```python
from build123d import *

# Parameters (mm, degrees)
F0_R     = 1.5
F0_W     = 114
F0_H     = 114
F0_W_2   = 110
F0_H_2   = 110
F1_DEPTH = 2
F0_W_3   = 7
F0_H_3   = 30
F2_DEPTH = 2.5
F0_H_4   = 5
F0_W_4   = 8
F3_DEPTH = 10
F4_SIZE  = 7.99999
F5_R     = 4
F6_DEPTH = 25
F7_R     = 3
F8_R     = 5
F10_D    = 3


# Not quite as in the source:
# - a fillet or chamfer is up to 0.001 mm smaller than in the source, because OpenCascade refuses the exact size


with BuildPart() as f1:
    # F0 (on Front) → F1 (new body)
    with BuildSketch(Plane.XZ):
        with BuildLine():
            Line((-68, 17.5), (-75, 17.5))
            Line((-75, 17.5), (-75, -17.5))
            Line((-75, -17.5), (-68, -17.5))
            Line((-68, -17.5), (-68, -56.2650060048))
            ThreePointArc((-68, -56.2650060048), (-60.8578643763, -60.8578643763), (-56.2650060048, -68))
            Line((-56.2650060048, -68), (56.2650060048, -68))
            ThreePointArc((56.2650060048, -68), (60.8578643763, -60.8578643763), (68, -56.2650060048))
            Line((68, -56.2650060048), (68, -20))
            Line((68, -20), (60, -20))
            Line((60, -20), (60, -15))
            Line((60, -15), (68, -15))
            Line((68, -15), (68, 15))
            Line((68, 15), (60, 15))
            Line((60, 15), (60, 20))
            Line((60, 20), (68, 20))
            Line((68, 20), (68, 56.2650060048))
            ThreePointArc((68, 56.2650060048), (60.8578643763, 60.8578643763), (56.2650060048, 68))
            Line((56.2650060048, 68), (-56.2650060048, 68))
            ThreePointArc((-56.2650060048, 68), (-60.8578643763, 60.8578643763), (-68, 56.2650060048))
            Line((-68, 56.2650060048), (-68, 17.5))
        make_face()
        with Locations((-70, 0)):
            Circle(F0_R, mode=Mode.SUBTRACT)
        Rectangle(F0_W, F0_H, mode=Mode.SUBTRACT)
        Rectangle(F0_W, F0_H)
        Rectangle(F0_W_2, F0_H_2, mode=Mode.SUBTRACT)
    extrude(amount=F1_DEPTH)

    # F0 (on Front) → F2 (join)
    with BuildSketch(Plane.XZ):
        with BuildLine():
            Line((-68, 68), (-68, 56.2650060048))
            ThreePointArc((-68, 56.2650060048), (-60.8578643763, 60.8578643763), (-56.2650060048, 68))
            Line((-56.2650060048, 68), (-68, 68))
        make_face()
        Polygon((75, 20), (75, 75), (-75, 75), (-75, 17.5), (-68, 17.5), (-68, 56.2650060048), (-68, 68), (-56.2650060048, 68), (56.2650060048, 68), (68, 68), (68, 56.2650060048), (68, 20), align=None)
        with BuildLine():
            ThreePointArc((56.2650060048, 68), (60.8578643763, 60.8578643763), (68, 56.2650060048))
            Line((68, 56.2650060048), (68, 68))
            Line((68, 68), (56.2650060048, 68))
        make_face()
        with BuildLine():
            Line((68, -68), (68, -56.2650060048))
            ThreePointArc((68, -56.2650060048), (60.8578643763, -60.8578643763), (56.2650060048, -68))
            Line((56.2650060048, -68), (68, -68))
        make_face()
        with BuildLine():
            ThreePointArc((-56.2650060048, -68), (-60.8578643763, -60.8578643763), (-68, -56.2650060048))
            Line((-68, -56.2650060048), (-68, -68))
            Line((-68, -68), (-56.2650060048, -68))
        make_face()
        Polygon((-68, -17.5), (-75, -17.5), (-75, -75), (75, -75), (75, -20), (68, -20), (68, -56.2650060048), (68, -68), (56.2650060048, -68), (-56.2650060048, -68), (-68, -68), (-68, -56.2650060048), align=None)
        with Locations((71.5, 0)):
            Rectangle(F0_W_3, F0_H_3)
    extrude(amount=F2_DEPTH)

    # F0 (on Front) → F3 (join)
    with BuildSketch(Plane.XZ):
        with Locations((71.5, 17.5)):
            Rectangle(F0_W_3, F0_H_4)
        with Locations((64, 17.5)):
            Rectangle(F0_W_4, F0_H_4)
        with Locations((64, -17.5)):
            Rectangle(F0_W_4, F0_H_4)
        with Locations((71.5, -17.5)):
            Rectangle(F0_W_3, F0_H_4)
    extrude(amount=F3_DEPTH)

    # F4 (size 8 in the source; OpenCascade refuses exactly that, so slightly less here)
    f4_edges = [f1.edges().sort_by_distance(p)[0] for p in [
        (60, -10, 17.5),
        (60, -10, -17.5),
    ]]
    chamfer(f4_edges, length=F4_SIZE)

    # F5
    f5_edges = [f1.edges().sort_by_distance(p)[0] for p in [
        (75, -10, 17.5),
        (75, -10, -17.5),
    ]]
    fillet(f5_edges, radius=F5_R)

    # F0 (on Front) → F6 (join)
    with BuildSketch(Plane.XZ):
        Rectangle(F0_W, F0_H)
        Rectangle(F0_W_2, F0_H_2, mode=Mode.SUBTRACT)
    extrude(amount=-F6_DEPTH)

    # F7
    f7_edges = [f1.edges().sort_by_distance(p)[0] for p in [
        (-55, 11.5, 55),
        (55, 11.5, 55),
        (55, 11.5, -55),
        (-55, 11.5, -55),
    ]]
    fillet(f7_edges, radius=F7_R)

    # F8
    f8_edges = [f1.edges().sort_by_distance(p)[0] for p in [
        (57, 12.5, 57),
        (57, 12.5, -57),
        (-57, 12.5, -57),
        (-57, 12.5, 57),
        (-75, -1.25, 75),
        (-75, -1.25, -75),
        (75, -1.25, -75),
        (75, -1.25, 75),
    ]]
    fillet(f8_edges, radius=F8_R)

    # F10 (through all)
    with Locations(Plane.XY.offset(20)):
        with Locations((71, -6)):
            Hole(F10_D / 2)


solid = f1.part
```
Part model, mm, in its own coordinate system. A direction names the side the tool comes from. Coordinates: 2 decimals unless noted, no trailing zeros. Order: outer loops, then holes, each group sorted by start corner. A loop starts at its lowest first (then second) coordinate and runs counter-clockwise, first axis right, second up. Notation, with made-up numbers: (-29.5, -6.75) -> (-14.5, -6.75) arc R29 ccw to (-14.5, 23.25) -> close; hole circle Ø5 at (7, -8.5). An arc over 180 degrees is marked (long way). Put each result on its own line as item: value. Start each with the question number.
(1) Band-saw the part on A-A (x = 24). Give the cut face in (y, z).
(2) Pin check, flat tips, straight feed: pin 1 Ø2.5 at (x, y) = (71, -6.5) entering from -Z; pin 2 Ø8 at (x, y) = (25, 10) entering from +Z; pin 3 Ø6 at (x, y) = (43, 16) entering from -Z. Stop position of each tip, or through.
(3) Mould opens along X. For faces 1 (the face through (-57, 12, -1)), 2 (the face through (-55.2, 25, 25.6)), 3 (the face through (73.859, -8.797, 17.535)), 4 (the face through (60.773, -2.246, 60.943)) say: pulls with the +X half, pulls with the -X half, needs draft (parallel to the pull), parting line crosses it, or undercut.
(4) Probe line 1 along X through (y, z) = (7.5, 41.5); line 2 along Y through (x, z) = (71, 17). List the from-to ranges inside material, lowest first. Write a range as [from, to].
(5) Band-saw the part on B-B (z = -29). Give the cut face in (x, y).
(6) Which spindle directions (+Z, -Z, +X, -X, +Y, -Y) get a long thin tool onto all of the face, cutting with end or side? Do faces 5 (the face through (-60.943, -2.246, 60.773)), 6 (the face through (-56, 13, -55)), 7 (the face through (71, -2.5, 0)), 8 (the face through (-1, 11, 55)), 9 (the face through (-68, 0, 1)). Say none if no direction does.
(7) Band-saw the part on D-D (z = 59). Give the cut face in (x, y).
(8) Band-saw the part on C-C (y = 19). Give the cut face in (x, z).
Determined:
1. outline: (-2.5, -75) -> (0, -75) -> (0, -57) -> (25, -57) -> (25, -55) -> (-2, -55) -> (-2, -68) -> (-2.5, -68) -> close; (-2.5, 68) -> (-2, 68) -> (-2, 55) -> (25, 55) -> (25, 57) -> (0, 57) -> (0, 75) -> (-2.5, 75) -> close
2. pin 1: stops at z = -20
2. pin 2: stops at z = 57
2. pin 3: stops at z = -57
3. face 1: pulls with the -X half
3. face 2: needs draft
3. face 3: pulls with the +X half
3. face 4: undercut
4. line 1: x = [-57, -55], [55, 57]
4. line 2: y = [-10, -7.5], [-4.5, 0]
5. outline: (-75, -2.5) -> (-68, -2.5) -> (-68, -2) -> (-55, -2) -> (-55, 25) -> (-57, 25) -> (-57, 0) -> (-75, 0) -> close; (55, -2) -> (68, -2) -> (68, -2.5) -> (75, -2.5) -> (75, 0) -> (57, 0) -> (57, 25) -> (55, 25) -> close
6. face 5: -Y
6. face 6: -Z, -X, +Y
6. face 7: +X, -X, -Y
6. face 8: +Y, -Y
6. face 9: +Y
7. outline: (-75, -2.5) -> (-63, -2.5) -> (-63, -2) -> (63, -2) -> (63, -2.5) -> (75, -2.5) -> (75, 0) -> (-75, 0) -> close
8. outline: (-57, -52) arc R5 ccw to (-52, -57) -> (52, -57) arc R5 ccw to (57, -52) -> (57, 52) arc R5 ccw to (52, 57) -> (-52, 57) arc R5 ccw to (-57, 52) -> close; hole (-55, -52) arc R3 ccw to (-52, -55) -> (52, -55) arc R3 ccw to (55, -52) -> (55, 52) arc R3 ccw to (52, 55) -> (-52, 55) arc R3 ccw to (-55, 52) -> close
